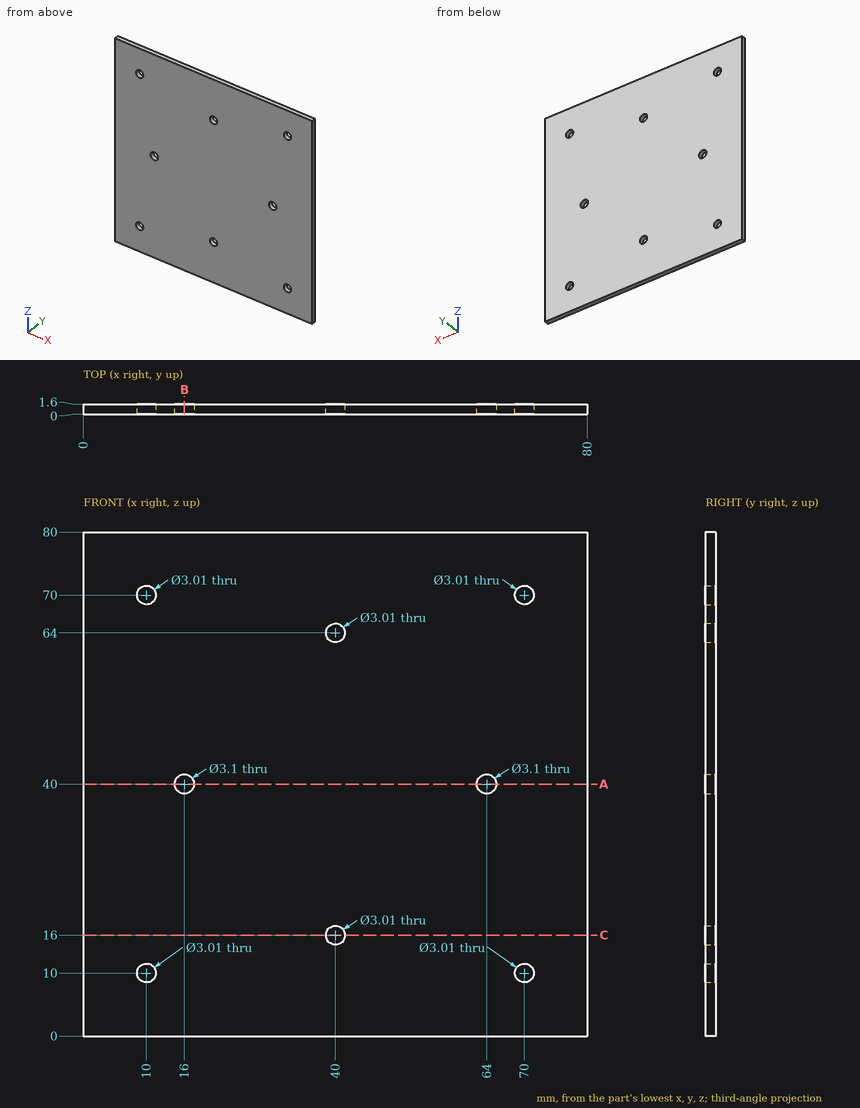
Source: three-view drawing plus pictorial views. Frame: mm from the lowest corner of the part. Round coordinates to 2 decimals unless told otherwise and drop trailing zeros. Loops run counter-clockwise (first coordinate to the right, second up) from the corner with the lowest first, then second, coordinate; pieces in that order, holes last.
1. Section query C-C on z = 16. Output: boundary loops of the cut face in (x, y) (3 decimals), and give its area (3 significant figures).
2. Section query B-B on x = 16. Output: boundary loops of the cut face in (y, z), and give its area (3 significant figures).
3. Section query A-A on z = 40. Output: boundary loops of the cut face in (x, y).
4. Ray query, L1, parallel to Z at x = 10, y = 1.15 (3 decimals); L2, parallel to X at y = 0.6, z = 64 (3 decimals). Return the intervals inside material, ascending.
Answers below:
1. outline: (0, 0) - (38.495, 0) - (38.495, 1.6) - (0, 1.6) - close; (41.505, 0) - (80, 0) - (80, 1.6) - (41.505, 1.6) - close
1. area: 123 mm2
2. outline: (0, 0) - (1.6, 0) - (1.6, 38.45) - (0, 38.45) - close; (0, 41.55) - (1.6, 41.55) - (1.6, 80) - (0, 80) - close
2. area: 123 mm2
3. outline: (0, 0) - (14.45, 0) - (14.45, 1.6) - (0, 1.6) - close; (17.55, 0) - (62.45, 0) - (62.45, 1.6) - (17.55, 1.6) - close; (65.55, 0) - (80, 0) - (80, 1.6) - (65.55, 1.6) - close
4. L1: z = 0 to 8.495, 11.505 to 68.495, 71.505 to 80
4. L2: x = 0 to 38.495, 41.505 to 80
